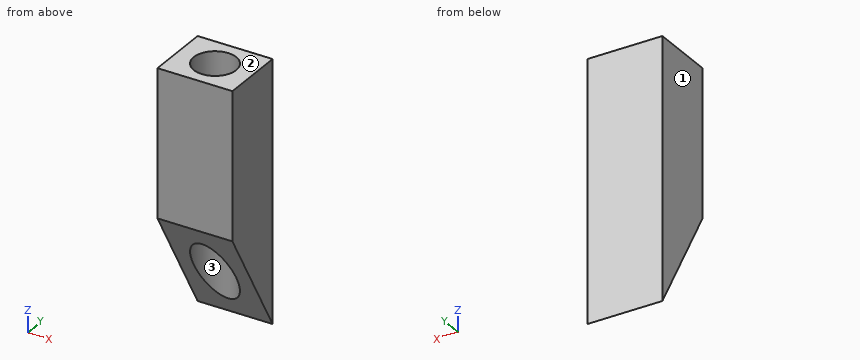
from build123d import *

# Parameters (mm, degrees)
SKETCH1_W           = 7.3406
SKETCH1_H           = 6.35
BOSS_EXTRUDE1_DEPTH = 25.4
CUT_EXTRUDE1_DEPTH  = 7.3406
SKETCH3_R           = 2.0828
CUT_EXTRUDE2_DEPTH  = 25.4


with BuildPart() as part:
    # Sketch1 → Boss-Extrude1 (new body)
    with BuildSketch(Plane.XY):
        Rectangle(SKETCH1_W, SKETCH1_H)
    extrude(amount=BOSS_EXTRUDE1_DEPTH)

    # Sketch2 → Cut-Extrude1 (cut)
    with BuildSketch(Plane(origin=(3.6703, 0, 0), x_dir=(0, 0, -1), z_dir=(1, 0, 0))):
        Polygon((0, 3.175), (-10.998522628, -3.175), (0, -3.175), align=None)
    extrude(amount=-CUT_EXTRUDE1_DEPTH, mode=Mode.SUBTRACT)

    # Sketch3 → Cut-Extrude2 (cut)
    with BuildSketch(Plane.XY.offset(25.4)):
        Circle(SKETCH3_R)
    extrude(amount=-CUT_EXTRUDE2_DEPTH, mode=Mode.SUBTRACT)


solid = part.part
Design review of the part built by this model. Coordinates are the model's own, in mm. Face numbers are marked on the shaded views. Give positions to 0.01 mm unless a question says otherwise; leave off trailing zeros. Loops run counter-clockwise (first coordinate to the right, second up) from the corner with the lowest first, then second, coordinate; pieces in that order, holes last. Notation, with made-up numbers: M 54.5,72.5 L 98.5,72.5 A12 cw 98.5,91.5 Z; hole C 13,-26 d4. An arc over 180 degrees is marked long. One line per question, with ' | ' between items. Start each with the question number.
1. Add section A-A (y = -1.25). Write out the cut boundary in (x, z).
2. Add section B-B (x = 1.75). Write out the cut boundary in (y, z) (3 decimals).
3. Insertion check: P1, Ø1.5, axis at x = 1.5, y = 0.5, coming from the +Z side. The pin has a flat end and moves straight along its axis. Give the tip position at first contact, or say it passes through.
4. To check wall thickness, follow L1, parallel to Y at x = 0, z = 17.5 (3 decimals); L2, parallel to X at y = 0, z = 9.5; L3, parallel to X at y = 0.75, z = 16.25. State the ranges of each line that lie inside material, in increasing order.
5. Add section D-D (x = -2.5). Write out the cut boundary in (y, z) (3 decimals).
6. The part is to be moulded in two halves that separate along X. For the marked faces 1, 2 and 3, say which applies: released by +X, released by -X, zero draft, split by the parting line, or undercut.
7. Add section C-C (z = 11.5). Write out the cut boundary in (x, y) (3 decimals), plus the area to 3 significant figures.
Worked out:
1) outline: M -3.67,7.66 L -1.67,7.66 L -1.67,25.4 L -3.67,25.4 Z; M 1.67,7.66 L 3.67,7.66 L 3.67,25.4 L 1.67,25.4 Z
2) outline: M -3.175,10.999 L -1.129,7.455 L -1.129,25.4 L -3.175,25.4 Z; M 1.129,3.543 L 3.175,0 L 3.175,25.4 L 1.129,25.4 Z
3) P1: stops at z = 25.4
4) L1: y = -3.175 to -2.083, 2.083 to 3.175 | L2: x = -3.67 to -2.08, 2.08 to 3.67 | L3: x = -3.67 to -1.94, 1.94 to 3.67
5) outline: M -3.175,10.999 L 3.175,0 L 3.175,25.4 L -3.175,25.4 Z
6) face 1: released by -X | face 2: zero draft | face 3: undercut
7) outline: M -3.67,-3.175 L 3.67,-3.175 L 3.67,3.175 L -3.67,3.175 Z; hole C 0,0 d4.166 | area: 33.0 mm²
